The listing builds one solid part. Answer for the finished solid, in the listing's coordinates (mm). A direction names the side the tool comes from. Round coordinates to 2 decimals unless told otherwise and drop trailing zeros. Order: outer loops, then holes, each group sorted by start corner. A loop starts at its lowest first (then second) coordinate and runs counter-clockwise, first axis right, second up. Notation, with made-up numbers: (24, 75.5) - (34, 75.5) arc R14 ccw to (34, 100.5) - close; hole circle Ø9 at (-34.75, -23.75). An arc over 180 degrees is marked (long way). Write item = value, one per line.
from build123d import *

# Parameters (mm, degrees)
F1_DEPTH      = 6
F2_R          = 0.75
F3_DEPTH      = 3
F3_DEPTH_BACK = 8
F4_R          = 2.99999
F5_R          = 2.99999
F6_R          = 2


# Not quite as in the source:
# - a fillet or chamfer is up to 0.001 mm smaller than in the source, because OpenCascade refuses the exact size


with BuildPart() as f1:
    # F0 (on Front) → F1 (new body)
    with BuildSketch(Plane.XZ):
        Polygon((5.5, 0), (0, 0), (0, -10), (16, -10), (16, 0), (10.5, 0), (10.5, 10), (5.5, 10), align=None)
    extrude(amount=F1_DEPTH)

    # F2 (on face) → F3 (join, two sides)
    with BuildSketch(Plane.YZ.offset(10.5)) as f3_sk:
        with Locations((-3, 6)):
            Circle(F2_R)
    extrude(amount=F3_DEPTH)
    extrude(f3_sk.sketch, amount=-F3_DEPTH_BACK)

    # F4 (radius 3 in the source; OpenCascade refuses exactly that, so slightly less here)
    f4_edges = [f1.edges().sort_by_distance(p)[0] for p in [
        (8, -6, 10),
        (8, 0, 10),
    ]]
    fillet(f4_edges, radius=F4_R)

    # F5 (radius 3 in the source; OpenCascade refuses exactly that, so slightly less here)
    f5_edges = [f1.edges().sort_by_distance(p)[0] for p in [
        (2.75, -6, 0),
        (2.75, 0, 0),
        (13.25, -6, 0),
        (13.25, 0, 0),
    ]]
    fillet(f5_edges, radius=F5_R)

    # F6
    f6_edges = [f1.edges().sort_by_distance(p)[0] for p in [
        (8, -6, -10),
        (8, 0, -10),
    ]]
    fillet(f6_edges, radius=F6_R)


solid = f1.part
Q1. For faces 1 (the face through (11.979, -3.595, 5.544)), 2 (the face through (8, 0, -2)), 3 (the face through (2.5, -3, 6)), determine the directions among +Z, -Z, +X, -X, +Y, -Y from which every point of the face is accessible in a straight line to the end or side of a thin tool.
Model answer:
face_1 = +X
face_2 = +Z, -Z, +X, -X, +Y
face_3 = +Z, -X, +Y, -Y
Q2. Section D-D on z = -1 is taken. Determine the outline of the cut face in (x, y), then the cut area to 3 significant figures.
Model answer:
outline = (0, -5.24) - (5.5, -5.24) - (5.5, -6) - (10.5, -6) - (10.5, -5.24) - (16, -5.24) - (16, -0.76) - (10.5, -0.76) - (10.5, 0) - (5.5, 0) - (5.5, -0.76) - (0, -0.76) - close
area = 79.2 mm^2
Q3. Find the intervals of material crossed by line 1 (X direction, y = -5.2, z = 6.5); line 2 (Z direction, x = 4.25, y = -3.5); line 3 (X direction, y = -3.1, z = 5.75), in increasing order. Write a range as from..to.
Model answer:
line_1 = 5.5..10.5
line_2 = -10..-0.04, 5.44..6.56
line_3 = 2.5..13.5
Q4. Section C-C on y = -1.55 is taken. Determine the outline of the cut face in (x, z), then the cut area to 3 significant figures.
Model answer:
outline = (0, -9.95) - (16, -9.95) - (16, -0.37) - (10.5, -0.37) - (10.5, 9.63) - (5.5, 9.63) - (5.5, -0.37) - (0, -0.37) - close
area = 203 mm^2
Q5. Flat-ended cylindrical pins translate along their axes: P1, Ø1.5, axis at y = -2.5, z = 6, coming from the -X side; P2, Ø3, axis at y = -3, z = 2, coming from the +X side; P3, Ø1.8, axis at y = -1.5, z = 2.5, coming from the -X side; P4, Ø2, axis at x = 5, y = -3, coming from the +Z side. Find the tip coordinate at first contact, or state that the pin passes through.
Model answer:
P1 = 2.5
P2 = 10.5
P3 = 5.5
P4 = 10
Q6. Determine the mould class of faces 4 (the face through (13.5, -3, 6)), 5 (the face through (7.96, -5.1, 9.14)), 6 (the face through (4.021, -3.595, 5.544)) for opening direction Z: released by +Z, released by -Z, zero draft, split by the parting line, or undercut.
Model answer:
face_4 = zero draft
face_5 = released by +Z
face_6 = undercut
Q7. Section B-B on z = 6 is taken. Determine the outline of the cut face in (x, y), then the cut area to 3 significant figures.
Model answer:
outline = (2.5, -3.75) - (5.5, -3.75) - (5.5, -6) - (10.5, -6) - (10.5, -3.75) - (13.5, -3.75) - (13.5, -2.25) - (10.5, -2.25) - (10.5, 0) - (5.5, 0) - (5.5, -2.25) - (2.5, -2.25) - close
area = 39.0 mm^2
